For this review, take the finished solid that the model builds, in its own axes (mm). Give positions to 0.01 mm unless a question says otherwise; leave off trailing zeros. Order: outer loops, then holes, each group sorted by start corner. A loop starts at its lowest first (then second) coordinate and runs counter-clockwise, first axis right, second up. Notation, with made-up numbers: (-5, 45) - (36, 45) arc R28 ccw to (36, 70) - close; hole circle Ø9 at (33.25, -31). An arc over 180 degrees is marked (long way). Use a Markdown table: item, result. Add a question column.
1) We need section C-C on x = 204.5. Write out the cut boundary in (y, z), then the cut area to 4 significant figures.
2) We need section D-D on x = 143. Write out the cut boundary in (y, z), then the cut area to 3 significant figures.
3) We need section B-B on y = -1.4. Give the number of separate pieces and of enclosed holes in the cut face, then the cut area to 3 significant figures.
4) Clearance check with flat-ended pins moving along their axes: P1, Ø1.5, axis at y = -2, z = 70.5, coming from the +X side; P2, Ø0.6, axis at x = 214, y = -2, coming from the +Z side; P3, Ø1.5, axis at y = -1.5, z = 76, coming from the +X side. State where each tip first meets the part, or that it passes through.
5) We need section A-A on x = 166.5. Write out the cut boundary in (y, z), then the cut area to 3 significant figures.
6) Wall thickness on L1, parallel to Z at x = 224, y = -1.35; L2, parallel to Z at x = 33, y = -2.3; L3, parallel to X at y = -1.35, z = 61: over which ranges is each line inside the solid? List them lowest first.
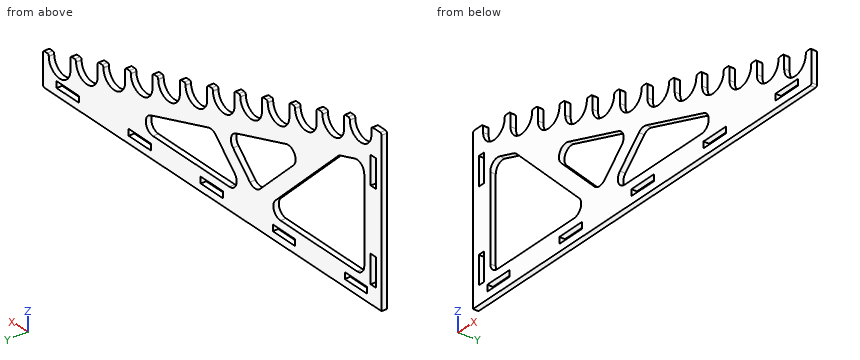
```python
from build123d import *

# Parameters (mm, degrees)
F1_DEPTH = 3
F2_R     = 1
F3_W     = 15.5
F3_H     = 3.5
F3_W_2   = 3.5
F3_H_2   = 15.5
F4_DEPTH = 25


with BuildPart() as f1:
    # F0 (on Front) → F1 (new body)
    with BuildSketch(Plane.XZ):
        with BuildLine():
            Line((0, 90), (0, 0))
            Line((0, 0), (235, 0))
            Line((235, 0), (235, 17.5337082297))
            ThreePointArc((235, 17.5337082297), (234.7071067812, 18.2408150109), (234, 18.5337082297))
            Line((234, 18.5337082297), (232, 18.5337082297))
            ThreePointArc((232, 18.5337082297), (231.2928932188, 18.2408150109), (231, 17.5337082297))
            Line((231, 17.5337082297), (231, 17.3050220176))
            ThreePointArc((231, 17.3050220176), (223.5, 9.8050220176), (216, 17.3050220176))
            Line((216, 17.3050220176), (216, 21.3050220176))
            Line((216, 21.3050220176), (216, 23.7787062281))
            ThreePointArc((216, 23.7787062281), (215.7071067812, 24.4858130093), (215, 24.7787062281))
            Line((215, 24.7787062281), (213, 24.7787062281))
            ThreePointArc((213, 24.7787062281), (212.2928932188, 24.4858130093), (212, 23.7787062281))
            Line((212, 23.7787062281), (212, 23.550020016))
            ThreePointArc((212, 23.550020016), (204.5, 16.050020016), (197, 23.550020016))
            Line((197, 23.550020016), (197, 27.550020016))
            Line((197, 27.550020016), (197, 30.0237042265))
            ThreePointArc((197, 30.0237042265), (196.7071067812, 30.7308110077), (196, 31.0237042265))
            Line((196, 31.0237042265), (194, 31.0237042265))
            ThreePointArc((194, 31.0237042265), (193.2928932188, 30.7308110077), (193, 30.0237042265))
            Line((193, 30.0237042265), (193, 29.7950180144))
            ThreePointArc((193, 29.7950180144), (185.5, 22.2950180144), (178, 29.7950180144))
            Line((178, 29.7950180144), (178, 33.7950180144))
            Line((178, 33.7950180144), (178, 36.2687022249))
            ThreePointArc((178, 36.2687022249), (177.7071067812, 36.9758090061), (177, 37.2687022249))
            Line((177, 37.2687022249), (175, 37.2687022249))
            ThreePointArc((175, 37.2687022249), (174.2928932188, 36.9758090061), (174, 36.2687022249))
            Line((174, 36.2687022249), (174, 36.0400160128))
            ThreePointArc((174, 36.0400160128), (166.5, 28.5400160128), (159, 36.0400160128))
            Line((159, 36.0400160128), (159, 40.0400160128))
            Line((159, 40.0400160128), (159, 42.5137002233))
            ThreePointArc((159, 42.5137002233), (158.7071067812, 43.2208070045), (158, 43.5137002233))
            Line((158, 43.5137002233), (156, 43.5137002233))
            ThreePointArc((156, 43.5137002233), (155.2928932188, 43.2208070045), (155, 42.5137002233))
            Line((155, 42.5137002233), (155, 42.2850140112))
            ThreePointArc((155, 42.2850140112), (147.5, 34.7850140112), (140, 42.2850140112))
            Line((140, 42.2850140112), (140, 46.2850140112))
            Line((140, 46.2850140112), (140, 48.7586982217))
            ThreePointArc((140, 48.7586982217), (139.7071067812, 49.4658050029), (139, 49.7586982217))
            Line((139, 49.7586982217), (137, 49.7586982217))
            ThreePointArc((137, 49.7586982217), (136.2928932188, 49.4658050029), (136, 48.7586982217))
            Line((136, 48.7586982217), (136, 48.5300120096))
            ThreePointArc((136, 48.5300120096), (128.5, 41.0300120096), (121, 48.5300120096))
            Line((121, 48.5300120096), (121, 52.5300120096))
            Line((121, 52.5300120096), (121, 55.0036962201))
            ThreePointArc((121, 55.0036962201), (120.7071067812, 55.7108030013), (120, 56.0036962201))
            Line((120, 56.0036962201), (118, 56.0036962201))
            ThreePointArc((118, 56.0036962201), (117.2928932188, 55.7108030013), (117, 55.0036962201))
            Line((117, 55.0036962201), (117, 54.775010008))
            ThreePointArc((117, 54.775010008), (109.5, 47.275010008), (102, 54.775010008))
            Line((102, 54.775010008), (102, 58.775010008))
            Line((102, 58.775010008), (102, 61.2451730918))
            ThreePointArc((102, 61.2451730918), (101.7058629727, 61.9535214974), (100.9964850724, 62.2451669144))
            Line((100.9964850724, 62.2451669144), (98.9964850724, 62.2381370157))
            ThreePointArc((98.9964850724, 62.2381370157), (98.2916515943, 61.9440061658), (98, 61.2381431931))
            Line((98, 61.2381431931), (98, 61.0200080064))
            ThreePointArc((98, 61.0200080064), (90.5, 53.5200080064), (83, 61.0200080064))
            Line((83, 61.0200080064), (83, 65.0200080064))
            Line((83, 65.0200080064), (83, 67.4936922169))
            ThreePointArc((83, 67.4936922169), (82.7071067812, 68.2007989981), (82, 68.4936922169))
            Line((82, 68.4936922169), (80, 68.4936922169))
            ThreePointArc((80, 68.4936922169), (79.2928932188, 68.2007989981), (79, 67.4936922169))
            Line((79, 67.4936922169), (79, 67.2650060048))
            ThreePointArc((79, 67.2650060048), (71.5, 59.7650060048), (64, 67.2650060048))
            Line((64, 67.2650060048), (64, 71.2650060048))
            Line((64, 71.2650060048), (64, 73.7351690886))
            ThreePointArc((64, 73.7351690886), (63.7058629727, 74.4435174942), (62.9964850724, 74.7351629112))
            Line((62.9964850724, 74.7351629112), (60.9964850724, 74.7281330125))
            ThreePointArc((60.9964850724, 74.7281330125), (60.2916515943, 74.4340021625), (60, 73.7281391899))
            Line((60, 73.7281391899), (60, 73.5100040032))
            ThreePointArc((60, 73.5100040032), (52.5, 66.0100040032), (45, 73.5100040032))
            Line((45, 73.5100040032), (45, 77.5100040032))
            Line((45, 77.5100040032), (45, 79.980167087))
            ThreePointArc((45, 79.980167087), (44.7058629727, 80.6885154926), (43.9964850724, 80.9801609096))
            Line((43.9964850724, 80.9801609096), (41.9964850724, 80.9731310109))
            ThreePointArc((41.9964850724, 80.9731310109), (41.2916515943, 80.6790001609), (41, 79.9731371883))
            Line((41, 79.9731371883), (41, 79.7550020016))
            ThreePointArc((41, 79.7550020016), (33.5, 72.2550020016), (26, 79.7550020016))
            Line((26, 79.7550020016), (26, 83.7550020016))
            Line((26, 83.7550020016), (26, 86.2251650854))
            ThreePointArc((26, 86.2251650854), (25.7058629727, 86.933513491), (24.9964850724, 87.225158908))
            Line((24.9964850724, 87.225158908), (22.9964850724, 87.2181290093))
            ThreePointArc((22.9964850724, 87.2181290093), (22.2916515943, 86.9239981593), (22, 86.2181351867))
            Line((22, 86.2181351867), (22, 86))
            ThreePointArc((22, 86), (14.5, 78.5), (7, 86))
            Line((7, 86), (7, 89))
            ThreePointArc((7, 89), (6.7071067812, 89.7071067812), (6, 90))
            Line((6, 90), (0, 90))
        make_face()
        with BuildLine():
            ThreePointArc((17, 12), (13.4644660941, 13.4644660941), (12, 17))
            Line((12, 17), (12, 63.5552642114))
            ThreePointArc((12, 63.5552642114), (14.0679569834, 67.6053412167), (18.5612494996, 68.3052642114))
            Line((18.5612494996, 68.3052642114), (28.2995777656, 65.1044304993))
            ThreePointArc((28.2995777656, 65.1044304993), (29.3580672309, 64.6131824005), (30.273862172, 63.8899644052))
            Line((30.273862172, 63.8899644052), (73.6282926713, 20.5355339059))
            ThreePointArc((73.6282926713, 20.5355339059), (74.7121564279, 15.0865828382), (70.0927587654, 12))
            Line((70.0927587654, 12), (17, 12))
        make_face(mode=Mode.SUBTRACT)
        with BuildLine():
            Line((103.0593050185, 32.8954784413), (91.3562147326, 21.1923881554))
            ThreePointArc((91.3562147326, 21.1923881554), (87.8206808267, 19.7279220614), (84.2851469208, 21.1923881554))
            Line((84.2851469208, 21.1923881554), (61.1221171694, 44.3554179068))
            ThreePointArc((61.1221171694, 44.3554179068), (60.3988991741, 50.5106907776), (66.2189005749, 52.6409518128))
            Line((66.2189005749, 52.6409518128), (101.0850206122, 41.1810123472))
            ThreePointArc((101.0850206122, 41.1810123472), (104.3875986483, 37.589969509), (103.0593050185, 32.8954784413))
        make_face(mode=Mode.SUBTRACT)
        with BuildLine():
            ThreePointArc((160.202611153, 21.75), (163.578466068, 16.209430585), (158.6413616534, 12))
            Line((158.6413616534, 12), (105.5486028881, 12))
            ThreePointArc((105.5486028881, 12), (100.9292052255, 15.0865828382), (102.0130689821, 20.5355339059))
            Line((102.0130689821, 20.5355339059), (115.1469251322, 33.669390056))
            ThreePointArc((115.1469251322, 33.669390056), (117.5235018764, 34.9976836858), (120.2437085377, 34.88385615))
            Line((120.2437085377, 34.88385615), (160.202611153, 21.75))
        make_face(mode=Mode.SUBTRACT)
    extrude(amount=F1_DEPTH)

    # F2
    f2_edges = [f1.edges().sort_by_distance(p)[0] for p in [
        (235, -1.5, 0),
        (0, -1.5, 90),
    ]]
    fillet(f2_edges, radius=F2_R)

    # F3 (on face) → F4 (cut)
    with BuildSketch(Plane.XZ.offset(3)):
        with Locations((17.75, 5.75)):
            Rectangle(F3_W, F3_H)
        with Locations((5.75, 17.75)):
            Rectangle(F3_W_2, F3_H_2)
        with Locations((5.75, 67.75)):
            Rectangle(F3_W_2, F3_H_2)
        with Locations((67.75, 5.75)):
            Rectangle(F3_W, F3_H)
        with Locations((117.75, 5.75)):
            Rectangle(F3_W, F3_H)
        with Locations((167.75, 5.75)):
            Rectangle(F3_W, F3_H)
        with Locations((217.75, 5.75)):
            Rectangle(F3_W, F3_H)
    extrude(amount=-F4_DEPTH, mode=Mode.SUBTRACT)


solid = f1.part
```
Checked values:
| question | item | result |
|---|---|---|
| 1 | outline | (-3, 0) - (0, 0) - (0, 16.05) - (-3, 16.05) - close |
| 1 | area | 48.15 mm² |
| 2 | outline | (-3, 0) - (0, 0) - (0, 12) - (-3, 12) - close; (-3, 27.4) - (0, 27.4) - (0, 36.29) - (-3, 36.29) - close |
| 2 | area | 62.6 mm² |
| 3 | separate pieces | 1 |
| 3 | enclosed holes | 10 |
| 3 | area | 6,930 mm² |
| 4 | P1 | x = 64 |
| 4 | P2 | z = 24.78 |
| 4 | P3 | x = 45 |
| 5 | outline | (-3, 0) - (0, 0) - (0, 4) - (-3, 4) - close; (-3, 7.5) - (0, 7.5) - (0, 28.54) - (-3, 28.54) - close |
| 5 | area | 75.1 mm² |
| 6 | L1 | 0 to 4, 7.5 to 9.82 |
| 6 | L2 | 0 to 12, 61.16 to 72.27 |
| 6 | L3 | 0 to 4, 7.5 to 12, 33.16 to 67.38, 75.62 to 83, 98 to 102 |
